Source: three-view drawing plus pictorial views. Frame: mm from the lowest corner of the part. A direction names the side the tool comes from. Give positions to 0.01 mm unless a question says otherwise; leave off trailing zeros. Order: outer loops, then holes, each group sorted by start corner. A loop starts at its lowest first (then second) coordinate and runs counter-clockwise, first axis right, second up.
1) Section A-A, the plane y = 1.7. Return loops of the section in (x, z), plus the area to 3 significant figures.
2) Section C-C, the plane z = 17. Return loops of the section in (x, y), plus the area to 3 significant figures.
3) Section B-B, the plane x = 11.5. Return loops of the section in (y, z).
4) Material intervals for line 1 (Z direction, x = 8, y = 1.7); line 2 (X direction, y = 3.25, z = 12), sorted ascending.
5) Access query for the marked faces 1 and 2. Directions: +Z, -Z, +X, -X, +Y, -Y. A direction counts if a zero-diameter tool reaches every point of the face in a straight line with its end or side. Return the directions, or none.
6) First-contact query: P1, Ø1.8, axis at y = 3.5, z = 23.5, coming from the -X side; P2, Ø0.6, axis at y = 1.5, z = 22.5, coming from the -X side; P3, Ø1.4, axis at x = 13, y = 2, coming from the -Z side; P4, Ø1.3, axis at y = 2, z = 16, coming from the +X side. Flat tips, straight axial feed; report the tip coordinate or a pass-through.
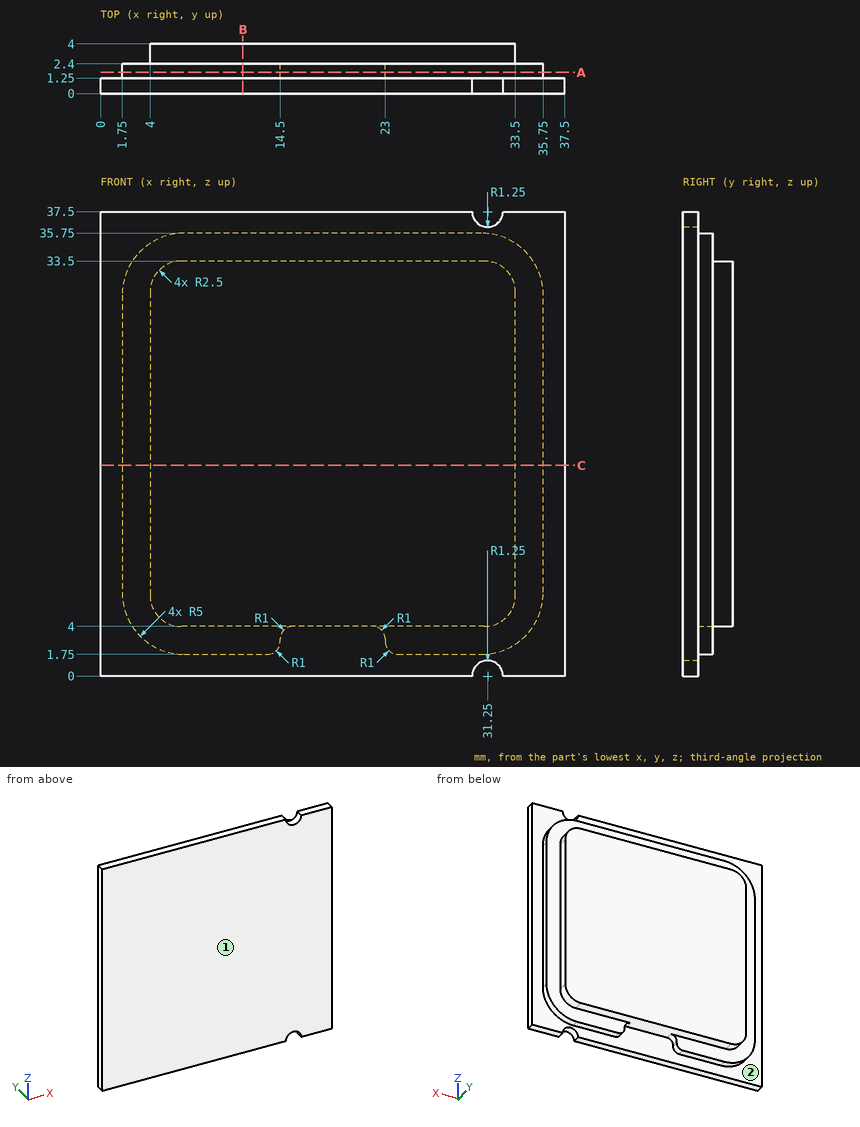
From the geometry:
1. outline: (1.75, 6.75) arc R5 ccw to (6.75, 1.75) - (13.5, 1.75) arc R1 ccw to (14.5, 2.75) - (14.5, 3) arc R1 cw to (15.5, 4) - (22, 4) arc R1 cw to (23, 3) - (23, 2.75) arc R1 ccw to (24, 1.75) - (30.75, 1.75) arc R5 ccw to (35.75, 6.75) - (35.75, 30.75) arc R5 ccw to (30.75, 35.75) - (6.75, 35.75) arc R5 ccw to (1.75, 30.75) - close
1. area: 1,120 mm2
2. outline: (0, 0) - (37.5, 0) - (37.5, 1.25) - (35.75, 1.25) - (35.75, 2.4) - (33.5, 2.4) - (33.5, 4) - (4, 4) - (4, 2.4) - (1.75, 2.4) - (1.75, 1.25) - (0, 1.25) - close
2. area: 133 mm2
3. outline: (0, 0) - (1.25, 0) - (1.25, 1.75) - (2.4, 1.75) - (2.4, 4) - (4, 4) - (4, 33.5) - (2.4, 33.5) - (2.4, 35.75) - (1.25, 35.75) - (1.25, 37.5) - (0, 37.5) - close
4. line 1: z = 1.75 to 35.75
4. line 2: x = 4 to 33.5
5. face 1: +Z, -Z, +X, -X, -Y
5. face 2: +Y
6. P1: stops at x = 4
6. P2: stops at x = 0
6. P3: stops at z = 1.75
6. P4: stops at x = 35.75
